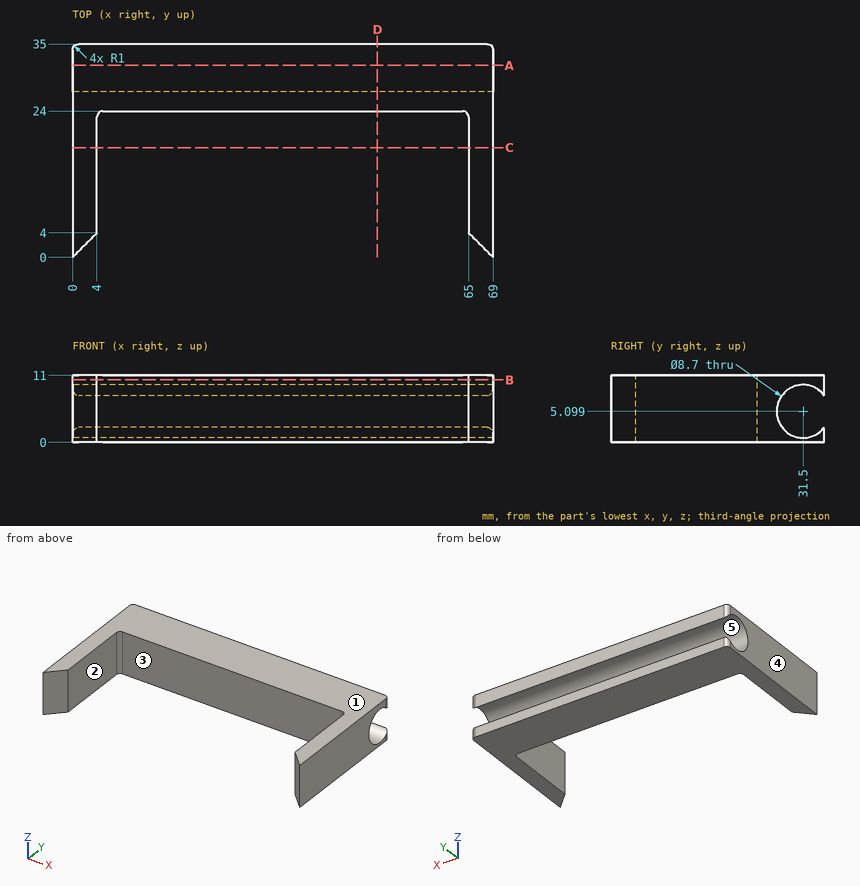
Drawing for the job (mm, zero at the part's lowest x, y, z). A direction names the side the tool comes from. Coordinates: 2 decimals unless noted, no trailing zeros. Loops run counter-clockwise (first coordinate to the right, second up) from the corner with the lowest first, then second, coordinate; pieces in that order, holes last. Notation, with made-up numbers: (-8, -37.5) - (50, -37.5) arc R26 cw to (50, -20.5) - close; hole circle Ø5 at (-27.75, 79). An arc over 180 degrees is marked (long way). Return JSON: item names as keys, results as strings.
1. Mould opens along Y. For the marked faces 3, 4 and 5 say: released by +Y, released by -Y, zero draft, split by the parting line, or undercut.
Result:
{"face 3": "released by -Y", "face 4": "zero draft", "face 5": "undercut"}
2. Band-saw the part on A-A (y = 31.5). Give the cut face in (x, z).
Result:
{"outline": "(0, 0) - (69, 0) - (69, 0.75) - (0, 0.75) - close; (0, 9.45) - (69, 9.45) - (69, 11) - (0, 11) - close"}
3. Drop a flat-ended pin along its axis: pin 1 (1.5 mm diameter, centred on x = 53, z = 2, fed in from -Y). Give the stop position or say it passes through.
Result:
{"pin 1": "stops at y = 24"}
4. Band-saw the part on D-D (x = 50). Give the cut face in (y, z).
Result:
{"outline": "(24, 0) - (35, 0) - (35, 2.52) arc R4.35 cw (long way) to (35, 7.68) - (35, 11) - (24, 11) - close"}
5. Probe L1, parallel to X at y = 5.5, z = 6.5; L2, parallel to Y at x = 17, z = 5; L3, parallel to Z at x = 36.5, y = 31.5. List the from-to ranges inside material, lowest first. Write a range as from..to.
Result:
{"L1": "x = 0..4, 65..69", "L2": "y = 24..27.15", "L3": "z = 0..0.75, 9.45..11"}
6. Band-saw the part on B-B (z = 10.25). Give the cut face in (x, y), and give its area (3 significant figures).
Result:
{"outline": "(0, 0) - (4, 4) - (4, 23) arc R1 cw to (5, 24) - (64, 24) arc R1 cw to (65, 23) - (65, 4) - (69, 0) - (69, 34) arc R1 ccw to (68, 35) - (1, 35) arc R1 ccw to (0, 34) - close", "area": "935 mm2"}
7. Band-saw the part on C-C (y = 18). Give the cut face in (x, z).
Result:
{"outline": "(0, 0) - (4, 0) - (4, 11) - (0, 11) - close; (65, 0) - (69, 0) - (69, 11) - (65, 11) - close"}
8. 3-axis set-ups, long thin cutter, end or side, ignore diameter. For the marked faces 1 and 2: which of +Z, -Z, +X, -X, +Y, -Y reach the whole face in a straight line?
Result:
{"face 1": "+Z, +X, -X, +Y, -Y", "face 2": "+Z, -Z, -Y"}
